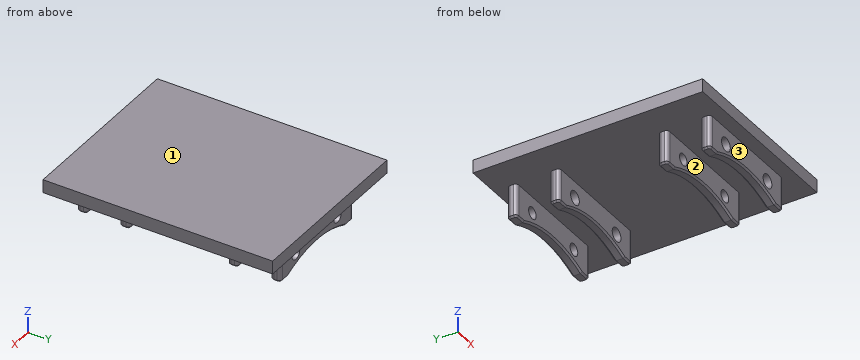
from build123d import *

# Parameters (mm, degrees)
SKETCH1_W               = 55
SKETCH1_H               = 70
BOSS_EXTRUDE1_DEPTH     = 4
BOSS_EXTRUDE2_DEPTH     = 10
SKETCH3_R               = 1.807722862
SKETCH3_R_2             = 1.85
CUT_EXTRUDE1_DEPTH      = 5
CUT_EXTRUDE1_DEPTH_BACK = 67
SKETCH4_R               = 2.1
CUT_EXTRUDE2_DEPTH      = 5
CUT_EXTRUDE2_DEPTH_BACK = 3
CUT_EXTRUDE3_START      = -46
SKETCH4_2_R             = 2.1
CUT_EXTRUDE3_DEPTH      = 3
CHAMFER1_SIZE           = 0.5
SKETCH5_R               = 33.04
CUT_EXTRUDE4_DEPTH      = 62
CHAMFER2_SIZE           = 0.5


with BuildPart() as part:
    # Sketch1 → Boss-Extrude1 (new body)
    with BuildSketch(Plane.XY):
        Rectangle(SKETCH1_W, SKETCH1_H)
    extrude(amount=BOSS_EXTRUDE1_DEPTH)

    # Sketch2 → Boss-Extrude2 (add)
    with BuildSketch(Plane(origin=(0, 0, 0), x_dir=(-1, 0, 0), z_dir=(0, 0, -1))):
        with BuildLine():
            Line((-16.5, 28), (16.5, 28))
            ThreePointArc((16.5, 28), (17.207106781, 28.292893219), (17.5, 29))
            Line((17.5, 29), (17.5, 30))
            ThreePointArc((17.5, 30), (17.207106781, 30.707106781), (16.5, 31))
            Line((16.5, 31), (-16.5, 31))
            ThreePointArc((-16.5, 31), (-17.207106781, 30.707106781), (-17.5, 30))
            Line((-17.5, 30), (-17.5, 29))
            ThreePointArc((-17.5, 29), (-17.207106781, 28.292893219), (-16.5, 28))
        make_face()
        with BuildLine():
            Line((-16.5, 18), (16.5, 18))
            ThreePointArc((16.5, 18), (17.207106781, 17.707106781), (17.5, 17))
            Line((17.5, 17), (17.5, 16))
            ThreePointArc((17.5, 16), (17.207106781, 15.292893219), (16.5, 15))
            Line((16.5, 15), (-16.5, 15))
            ThreePointArc((-16.5, 15), (-17.207106781, 15.292893219), (-17.5, 16))
            Line((-17.5, 16), (-17.5, 17))
            ThreePointArc((-17.5, 17), (-17.207106781, 17.707106781), (-16.5, 18))
        make_face()
        with BuildLine():
            Line((-16.5, -31), (16.5, -31))
            ThreePointArc((16.5, -31), (17.207106781, -30.707106781), (17.5, -30))
            Line((17.5, -30), (17.5, -29))
            ThreePointArc((17.5, -29), (17.207106781, -28.292893219), (16.5, -28))
            Line((16.5, -28), (-16.5, -28))
            ThreePointArc((-16.5, -28), (-17.207106781, -28.292893219), (-17.5, -29))
            Line((-17.5, -29), (-17.5, -30))
            ThreePointArc((-17.5, -30), (-17.207106781, -30.707106781), (-16.5, -31))
        make_face()
        with BuildLine():
            Line((-16.5, -15), (16.5, -15))
            ThreePointArc((16.5, -15), (17.207106781, -15.292893219), (17.5, -16))
            Line((17.5, -16), (17.5, -17))
            ThreePointArc((17.5, -17), (17.207106781, -17.707106781), (16.5, -18))
            Line((16.5, -18), (-16.5, -18))
            ThreePointArc((-16.5, -18), (-17.207106781, -17.707106781), (-17.5, -17))
            Line((-17.5, -17), (-17.5, -16))
            ThreePointArc((-17.5, -16), (-17.207106781, -15.292893219), (-16.5, -15))
        make_face()
    extrude(amount=BOSS_EXTRUDE2_DEPTH)

    # Sketch3 → Cut-Extrude1 (cut, two sides)
    with BuildSketch(Plane.XZ.offset(31)) as cut_extrude1_sk:
        with Locations((-10, -5)):
            Circle(SKETCH3_R)
        with Locations((10, -5)):
            Circle(SKETCH3_R_2)
    extrude(amount=CUT_EXTRUDE1_DEPTH, mode=Mode.SUBTRACT)
    extrude(cut_extrude1_sk.sketch, amount=-CUT_EXTRUDE1_DEPTH_BACK, mode=Mode.SUBTRACT)

    # Sketch4 → Cut-Extrude2 (cut, two sides)
    with BuildSketch(Plane.XZ.offset(31)) as cut_extrude2_sk:
        with Locations((10, -5)):
            Circle(SKETCH4_R)
        with Locations((-10, -5)):
            Circle(SKETCH4_R)
    extrude(amount=CUT_EXTRUDE2_DEPTH, mode=Mode.SUBTRACT)
    extrude(cut_extrude2_sk.sketch, amount=-CUT_EXTRUDE2_DEPTH_BACK, mode=Mode.SUBTRACT)

    # Sketch4<2> → Cut-Extrude3 (cut)
    with BuildSketch(Plane.XZ.offset(31).offset(CUT_EXTRUDE3_START)):
        with Locations((10, -5)):
            Circle(SKETCH4_2_R)
        with Locations((-10, -5)):
            Circle(SKETCH4_2_R)
    extrude(amount=-CUT_EXTRUDE3_DEPTH, mode=Mode.SUBTRACT)

    # Chamfer1
    chamfer1_edges = [part.edges().sort_by_distance(p)[0] for p in [
        (17.207106781, 17.707106781, -10),
        (17.5, 16.5, -10),
        (17.207106781, 15.292893219, -10),
        (0, 15, -10),
        (-17.207106781, 15.292893219, -10),
        (-17.5, 16.5, -10),
        (-17.207106781, 17.707106781, -10),
        (0, 18, -10),
        (-17.207106781, 30.707106781, -10),
        (0, 31, -10),
        (17.207106781, 30.707106781, -10),
        (17.5, 29.5, -10),
        (17.207106781, 28.292893219, -10),
        (0, 28, -10),
        (-17.207106781, 28.292893219, -10),
        (-17.5, 29.5, -10),
        (-17.207106781, -30.707106781, -10),
        (-17.5, -29.5, -10),
        (-17.207106781, -28.292893219, -10),
        (0, -28, -10),
        (17.207106781, -28.292893219, -10),
        (17.5, -29.5, -10),
        (17.207106781, -30.707106781, -10),
        (0, -31, -10),
        (-17.207106781, -15.292893219, -10),
        (0, -15, -10),
        (17.207106781, -15.292893219, -10),
        (17.5, -16.5, -10),
        (17.207106781, -17.707106781, -10),
        (0, -18, -10),
        (-17.207106781, -17.707106781, -10),
        (-17.5, -16.5, -10),
    ]]
    chamfer(chamfer1_edges, length=CHAMFER1_SIZE)

    # Sketch5 → Cut-Extrude4 (cut)
    with BuildSketch(Plane(origin=(0, 31, 0), x_dir=(1, 0, 0), z_dir=(0, 1, 0))):
        with Locations((0, 40)):
            Circle(SKETCH5_R)
    extrude(amount=-CUT_EXTRUDE4_DEPTH, mode=Mode.SUBTRACT)

    # Chamfer2
    chamfer2_edges = [part.edges().sort_by_distance(p)[0] for p in [
        (0, -31, -6.96),
        (0, -28, -6.96),
        (0, -18, -6.96),
        (0, -15, -6.96),
        (0, 15, -6.96),
        (0, 18, -6.96),
        (0, 28, -6.96),
        (0, 31, -6.96),
    ]]
    chamfer(chamfer2_edges, length=CHAMFER2_SIZE)


solid = part.part
The model under review builds one solid part; all positions refer to its coordinate system, in mm. Face numbers are marked on the shaded views. Round coordinates to 2 decimals unless told otherwise and drop trailing zeros. Order: outer loops, then holes, each group sorted by start corner. A loop starts at its lowest first (then second) coordinate and runs counter-clockwise, first axis right, second up. Notation, with made-up numbers: (-19, 68.25) -> (14, 68.25) arc R23 cw to (14, 82.25) -> close; hole circle Ø5 at (-17.75, 27). An arc over 180 degrees is marked (long way). Write item = value, one per line. Start each with the question number.
Item 1: Consider section A-A on z = -1.75. Count the separate pieces of the cut face and the enclosed holes in it, plus the area to 3 significant figures.
Item 2: Consider section B-B on x = 15.5. Write out the cut boundary in (y, z).
Item 3: Clearance check with flat-ended pins moving along their axes: pin 1 Ø1.1 at (y, z) = (-16.5, -4) entering from -X; pin 2 Ø6 at (x, y) = (4, 28) entering from -Z; pin 3 Ø5.5 at (x, z) = (-10, -5) entering from +Y. State where each tip first meets the part, or that it passes through.
Item 4: For line 1 along Y through (x, z) = (0, -5); line 2 along X through (y, z) = (-17, -2.75); line 3 along Z through (x, y) = (14, 1), list the stretches that pass through material, from the lowest coordinate up.
Item 5: Mouldability with a two-part tool opening along Y and no side actions: class the marked faces 1, 2 and 3 as released by +Y, released by -Y, zero draft, split by the parting line, or undercut.
Conclusion:
q1.separate_pieces = 4
q1.enclosed_holes = 0
q1.area = 417 mm2
q2.outline = (-35, 0) -> (-31, 0) -> (-31, -9.5) -> (-30.5, -10) -> (-28.5, -10) -> (-28, -9.5) -> (-28, 0) -> (-18, 0) -> (-18, -9.5) -> (-17.5, -10) -> (-15.5, -10) -> (-15, -9.5) -> (-15, 0) -> (15, 0) -> (15, -9.5) -> (15.5, -10) -> (17.5, -10) -> (18, -9.5) -> (18, 0) -> (28, 0) -> (28, -9.5) -> (28.5, -10) -> (30.5, -10) -> (31, -9.5) -> (31, 0) -> (35, 0) -> (35, 4) -> (-35, 4) -> close
q3.pin_1 = -17.5
q3.pin_2 = -7.7
q3.pin_3 = 31
q4.line_1 = -31 to -28, -18 to -15, 15 to 18, 28 to 31
q4.line_2 = -17.5 to 17.5
q4.line_3 = 0 to 4
q5.face_1 = zero draft
q5.face_2 = undercut
q5.face_3 = released by -Y
